Autodesk Fusion 360 part; units mm, degrees
sketch "Sketch1" plane through (-0.0003, 0, -14.0546) normal (0, 0, 1) x (0, 1, 0)
  arc A0 (15.0114, -7.5039) -> (14.5034, -6.9959) centre (14.5034, -7.5039) ccw
  line L0 (15.0114, -7.5039) -> (15.0114, -11.1107)
  arc A1 (14.5034, -11.6187) -> (15.0114, -11.1107) centre (14.5034, -11.1107) ccw
  line L1 (14.5034, -11.6187) -> (10.8966, -11.6187)
  arc A2 (10.3886, -11.1107) -> (10.8966, -11.6187) centre (10.8966, -11.1107) ccw
  line L2 (10.3886, -11.1107) -> (10.3886, -7.5039)
  arc A3 (10.8966, -6.9959) -> (10.3886, -7.5039) centre (10.8966, -7.5039) ccw
  line L3 (10.8966, -6.9959) -> (14.5034, -6.9959)
  arc A4 (27.7114, -7.5039) -> (27.2034, -6.9959) centre (27.2034, -7.5039) ccw
  line L4 (27.7114, -7.5039) -> (27.7114, -11.1107)
  arc A5 (27.2034, -11.6187) -> (27.7114, -11.1107) centre (27.2034, -11.1107) ccw
  line L5 (27.2034, -11.6187) -> (23.5966, -11.6187)
  arc A6 (23.0886, -11.1107) -> (23.5966, -11.6187) centre (23.5966, -11.1107) ccw
  line L6 (23.0886, -11.1107) -> (23.0886, -7.5039)
  arc A7 (23.5966, -6.9959) -> (23.0886, -7.5039) centre (23.5966, -7.5039) ccw
  line L7 (23.5966, -6.9959) -> (27.2034, -6.9959)
  arc A8 (40.4114, -7.5039) -> (39.9034, -6.9959) centre (39.9034, -7.5039) ccw
  line L8 (40.4114, -7.5039) -> (40.4114, -11.1107)
  arc A9 (39.9034, -11.6187) -> (40.4114, -11.1107) centre (39.9034, -11.1107) ccw
  line L9 (39.9034, -11.6187) -> (36.2966, -11.6187)
  arc A10 (35.7886, -11.1107) -> (36.2966, -11.6187) centre (36.2966, -11.1107) ccw
  line L10 (35.7886, -11.1107) -> (35.7886, -7.5039)
  arc A11 (36.2966, -6.9959) -> (35.7886, -7.5039) centre (36.2966, -7.5039) ccw
  line L11 (36.2966, -6.9959) -> (39.9034, -6.9959)
  arc A12 (53.1114, -7.5039) -> (52.6034, -6.9959) centre (52.6034, -7.5039) ccw
  line L12 (53.1114, -7.5039) -> (53.1114, -11.1107)
  arc A13 (52.6034, -11.6187) -> (53.1114, -11.1107) centre (52.6034, -11.1107) ccw
  line L13 (52.6034, -11.6187) -> (48.9966, -11.6187)
  arc A14 (48.4886, -11.1107) -> (48.9966, -11.6187) centre (48.9966, -11.1107) ccw
  line L14 (48.4886, -11.1107) -> (48.4886, -7.5039)
  arc A15 (48.9966, -6.9959) -> (48.4886, -7.5039) centre (48.9966, -7.5039) ccw
  line L15 (48.9966, -6.9959) -> (52.6034, -6.9959)
  arc A16 (65.8114, -7.5039) -> (65.3034, -6.9959) centre (65.3034, -7.5039) ccw
  line L16 (65.8114, -7.5039) -> (65.8114, -11.1107)
  arc A17 (65.3034, -11.6187) -> (65.8114, -11.1107) centre (65.3034, -11.1107) ccw
  line L17 (65.3034, -11.6187) -> (61.6966, -11.6187)
  arc A18 (61.1886, -11.1107) -> (61.6966, -11.6187) centre (61.6966, -11.1107) ccw
  line L18 (61.1886, -11.1107) -> (61.1886, -7.5039)
  arc A19 (61.6966, -6.9959) -> (61.1886, -7.5039) centre (61.6966, -7.5039) ccw
  line L19 (61.6966, -6.9959) -> (65.3034, -6.9959)
  arc A20 (2.3114, -7.5039) -> (1.8034, -6.9959) centre (1.8034, -7.5039) ccw
  line L20 (2.3114, -7.5039) -> (2.3114, -11.1107)
  arc A21 (1.8034, -11.6187) -> (2.3114, -11.1107) centre (1.8034, -11.1107) ccw
  line L21 (1.8034, -11.6187) -> (-1.8034, -11.6187)
  arc A22 (-2.3114, -11.1107) -> (-1.8034, -11.6187) centre (-1.8034, -11.1107) ccw
  line L22 (-2.3114, -11.1107) -> (-2.3114, -7.5039)
  arc A23 (-1.8034, -6.9959) -> (-2.3114, -7.5039) centre (-1.8034, -7.5039) ccw
  line L23 (-1.8034, -6.9959) -> (1.8034, -6.9959)
  line L24 (69.85, -15.6573) -> (69.85, -4.1003)
  line L25 (69.85, -4.1003) -> (58.1488, -4.1003)
  line L26 (58.1488, -4.1003) -> (57.15, -5.0991)
  line L27 (57.15, -5.0991) -> (56.1512, -4.1003)
  line L28 (56.1512, -4.1003) -> (-6.35, -4.1003)
  line L29 (-6.35, -4.1003) -> (-6.35, -13.1692)
  arc A24 (-6.35, -13.1692) -> (-6.2036, -13.5228) centre (-5.85, -13.1692) ccw
  line L30 (-6.2036, -13.5228) -> (-4.2155, -15.5109)
  arc A25 (-4.2155, -15.5109) -> (-3.8619, -15.6573) centre (-3.8619, -15.1573) ccw
  line L31 (-3.8619, -15.6573) -> (54.6619, -15.6573)
  arc A26 (54.6619, -15.6573) -> (55.0155, -15.5109) centre (54.6619, -15.1573) ccw
  line L32 (55.0155, -15.5109) -> (56.7964, -13.7299)
  arc A27 (57.5036, -13.7299) -> (56.7964, -13.7299) centre (57.15, -14.0834) ccw
  line L33 (57.5036, -13.7299) -> (59.2845, -15.5109)
  arc A28 (59.2845, -15.5109) -> (59.6381, -15.6573) centre (59.6381, -15.1573) ccw
  line L34 (59.6381, -15.6573) -> (69.85, -15.6573)
  line L35 (69.85, -6.6403) -> (69.85, -26.9603)
  line L36 (67.31, -29.5003) -> (46.99, -29.5003)
  line L37 (44.45, -26.9603) -> (44.45, -6.6403)
  line L38 (46.99, -4.1003) -> (67.31, -4.1003)
  arc A29 (46.99, -4.1003) -> (44.45, -6.6403) centre (46.99, -6.6403) ccw
  arc A30 (69.85, -6.6403) -> (67.31, -4.1003) centre (67.31, -6.6403) ccw
  arc A31 (67.31, -29.5003) -> (69.85, -26.9603) centre (67.31, -26.9603) ccw
  arc A32 (44.45, -26.9603) -> (46.99, -29.5003) centre (46.99, -26.9603) ccw
  line L39 (69.85, -15.6573) -> (69.85, -22.0073)
  line L40 (69.85, -22.0073) -> (44.45, -22.0073)
  line L41 (69.85, -22.0073) -> (61.9125, -22.0073)
  circle A33 centre (61.9125, -22.0073) radius 2.3813
  line L42 (61.9125, -22.0073) -> (52.3875, -22.0073)
  circle A34 centre (52.3875, -22.0073) radius 2.3813
  point P0 (69.85, -4.1003)
  point P1 (69.85, -29.5003)
  point P2 (44.45, -29.5003)
  point P3 (44.45, -4.1003)
  dimension "d1" = 25.4
  dimension "d2" = 25.4
  dimension "d3" = 25.4
  dimension "d4" = 2.54
  dimension "d5" = 6.35
  dimension "d6" = 7.9375
  dimension "d7" = 4.7625
  dimension "d8" = 9.525
  dimension "d9" = 4.7625
extrude "Extrude1" add sketch "Sketch1" along normal blind 3.9688 contours L24 L25 L26 L27 L28 L31 A26 L32 A27 L33 A28 L34 L35 L37 L38 A29 A30 | L31 A26 L32 A27 L33 A28 L34 L35 L37 L39 L40 L41 A33 L42 A34 | L35 L36 L37 A31 A32 L40 L41 A33 L42 A34 | L26 L27 L38
equation "d5 = ( 1 / 4 ) * 1 in"
equation "d6 = ( 5 / 16 ) * 1 in"
equation "d7 = ( 3 / 16 ) * 1 in"
equation "d8 = ( 3 / 8 ) * 1 in"
equation "d9 = ( 3 / 16 ) * 1 in"
equation "d10 = ( 5 / 32 ) * 1 in"
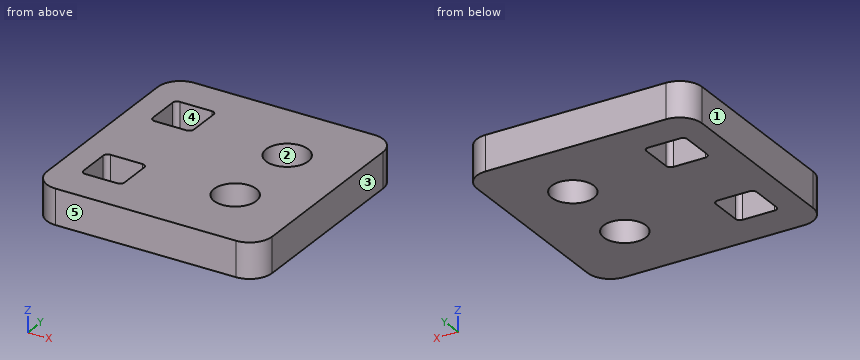
Geometry: final body of the model. Coordinates: model frame, mm. Face numbers are marked on the shaded views. A direction names the side the tool comes from. Round coordinates to 2 decimals unless told otherwise and drop trailing zeros. Loops run counter-clockwise (first coordinate to the right, second up) from the corner with the lowest first, then second, coordinate; pieces in that order, holes last. Notation, with made-up numbers: (10.5, 68) -> (43.5, 68) arc R19 cw to (43.5, 73) -> close; hole circle Ø5 at (41, -6.75). An arc over 180 degrees is marked (long way). One line per question, with ' | ' between items. Start each with the question number.
1. Set-up query: the marked faces 4 and 5. Return all of +Z, -Z, +X, -X, +Y, -Y with unobstructed straight access to the full face (end or side cutting, diameter ignored); none if empty.
2. Section B-B on z = -13.2. Output: boundary loops of the cut face in (x, y).
3. Mould query, pull axis X, two halves, no side actions, for the marked faces 1, 2 and 3. Classes: pulls with the +X half, pulls with the -X half, needs draft (parallel to the pull), parting line crosses it, or undercut.
4. Section A-A on y = 65. Output: boundary loops of the cut face in (x, z), and give its area (3 significant figures).
5. Line query: line 1 along Y through (x, z) = (7.75, -12.15); line 2 along Y through (x, z) = (23.5, -10.75); line 3 along Y through (x, z) = (6.5, -12.4). Output: solid intervals per line, ascending. Write a range as [from, to].
6. Contact query for a flat-ended pin moving along its axis: pin 1 (7.5 mm diameter, centred on x = 22.01, y = 61.91, fed in from +Z). Output: stop coordinate, or through.
7. Section C-C on y = 62. Output: boundary loops of the cut face in (x, z), and give its area (3 significant figures).
8. Section D-D on x = 20. Output: boundary loops of the cut face in (y, z), and give its area (3 significant figures).
Returned:
1) face 4: +Z, -Z | face 5: +Z, -Z, +X, -X, -Y
2) outline: (4.1, 46.99) arc R2.54 ccw to (6.64, 44.45) -> (26.96, 44.45) arc R2.54 ccw to (29.5, 46.99) -> (29.5, 67.31) arc R2.54 ccw to (26.96, 69.85) -> (6.64, 69.85) arc R2.54 ccw to (4.1, 67.31) -> close; hole (7, 49) arc R0.51 ccw to (7.5, 48.49) -> (11.11, 48.49) arc R0.51 ccw to (11.62, 49) -> (11.62, 52.6) arc R0.51 ccw to (11.11, 53.11) -> (7.5, 53.11) arc R0.51 ccw to (7, 52.6) -> close; hole (7, 61.7) arc R0.51 ccw to (7.5, 61.19) -> (11.11, 61.19) arc R0.51 ccw to (11.62, 61.7) -> (11.62, 65.3) arc R0.51 ccw to (11.11, 65.81) -> (7.5, 65.81) arc R0.51 ccw to (7, 65.3) -> close; hole circle Ø4.76 at (22.01, 52.39); hole circle Ø4.76 at (22.01, 61.91)
3) face 1: pulls with the -X half | face 2: undercut | face 3: pulls with the +X half
4) outline: (4.1, -14.05) -> (7, -14.05) -> (7, -10.09) -> (4.1, -10.09) -> close; (11.62, -14.05) -> (29.5, -14.05) -> (29.5, -10.09) -> (11.62, -10.09) -> close | area: 82.5 mm2
5) line 1: y = [44.45, 48.49], [53.11, 61.19], [65.81, 69.85] | line 2: y = [44.45, 50.53], [54.24, 60.06], [63.77, 69.85] | line 3: y = [44.45, 69.85]
6) pin 1: stops at z = -10.09
7) outline: (4.1, -14.05) -> (7, -14.05) -> (7, -10.09) -> (4.1, -10.09) -> close; (11.62, -14.05) -> (19.63, -14.05) -> (19.63, -10.09) -> (11.62, -10.09) -> close; (24.39, -14.05) -> (29.5, -14.05) -> (29.5, -10.09) -> (24.39, -10.09) -> close | area: 63.6 mm2
8) outline: (44.45, -14.05) -> (51.11, -14.05) -> (51.11, -10.09) -> (44.45, -10.09) -> close; (53.67, -14.05) -> (60.63, -14.05) -> (60.63, -10.09) -> (53.67, -10.09) -> close; (63.19, -14.05) -> (69.85, -14.05) -> (69.85, -10.09) -> (63.19, -10.09) -> close | area: 80.5 mm2
